Geometry check sheet. Reference: drawing and pictorial views, mm from the part's lowest x, y, z. A direction names the side the tool comes from. Coordinates: 2 decimals unless noted, no trailing zeros. Write each loop counter-clockwise with the first axis right and the second up, starting at its lowest first coordinate (ties: lowest second). Pieces come first, ordered by that corner, then holes. Notation, with made-up numbers: (65.5, 3) -> (95.5, 3) arc R17 cw to (95.5, 16) -> close; hole circle Ø11 at (73.5, 42.25). An arc over 180 degrees is marked (long way). Answer in a Markdown table with one row per item.
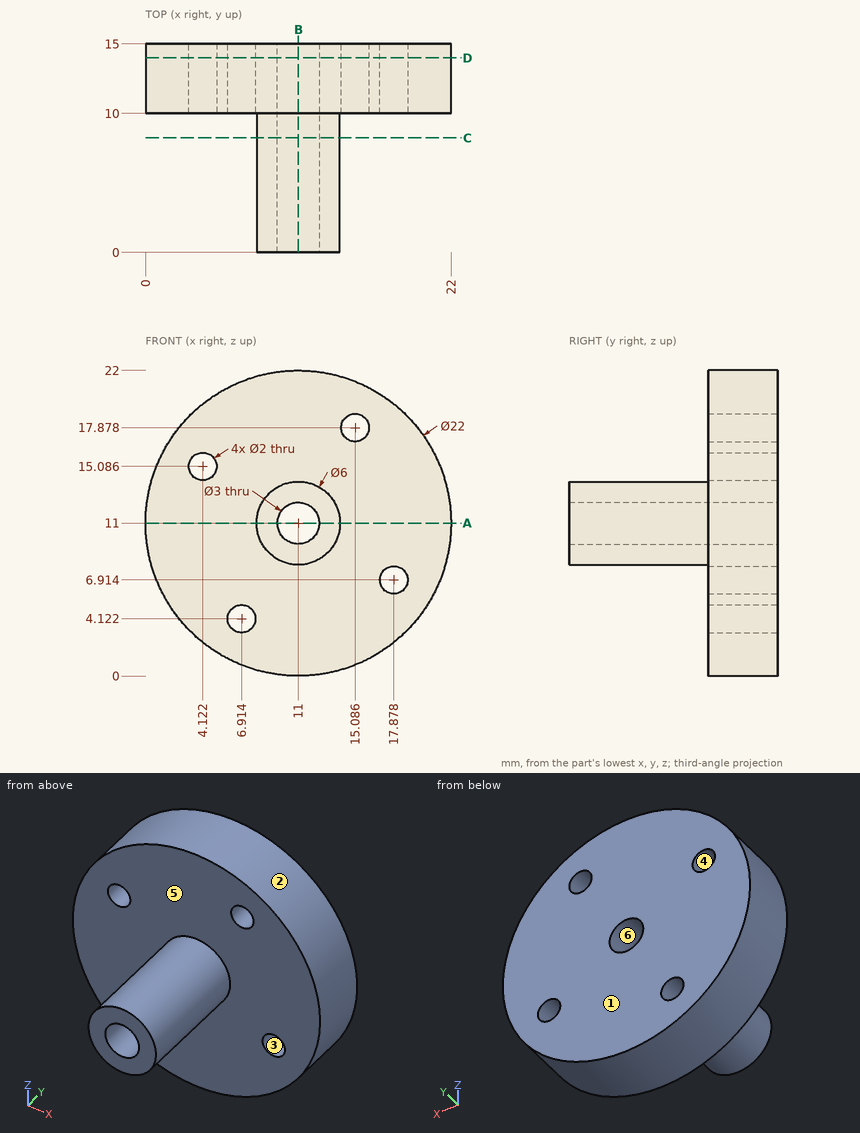
1. Thickness scan on line 1 (Z direction, x = 11, y = 11.75); line 2 (Y direction, x = 1.75, z = 6.5); line 3 (X direction, y = 4.5, z = 11.5) (1 decimal). Record the ranges inside material, lowest first. Write a range as from..to.
Geometry says:
| item | result |
|---|---|
| line 1 | 0..9.5, 12.5..22 |
| line 2 | 10..15 |
| line 3 | 8..9.6, 12.4..14 |
2. Mould release check, pull along X, two halves, no side actions. Record for the marked faces 1, 2, 3 and 4: released by +X, released by -X, zero draft, split by the parting line, or undercut.
Geometry says:
| item | result |
|---|---|
| face 1 | zero draft |
| face 2 | split by the parting line |
| face 3 | undercut |
| face 4 | undercut |
3. Tool access check on the marked faces 5 and 6. Record the directions out of +Z, -Z, +X, -X, +Y, -Y that give a thin tool (end or side, any length) a straight path to the whole face; none if there is none.
Geometry says:
| item | result |
|---|---|
| face 5 | -Y |
| face 6 | +Y, -Y |
4. Depth check by flat-ended pin: P1, Ø3, axis at y = 12, z = 13.5, coming from the +X side; P2, Ø2.5, axis at x = 6.91, z = 4.12, coming from the -Y side; P3, Ø1.5, axis at y = 4, z = 13, coming from the -X side. Enter the tip coordinate at first touch or a pass-through.
Geometry says:
| item | result |
|---|---|
| P1 | x = 21.95 |
| P2 | y = 10 |
| P3 | x = 8.27 |
5. Section check D-D, the plane y = 14. Record the boundary of the cut face in (x, z).
Geometry says:
| item | result |
|---|---|
| outline | circle Ø22 at (11, 11); hole circle Ø2 at (4.12, 15.09); hole circle Ø2 at (6.91, 4.12); hole circle Ø3 at (11, 11); hole circle Ø2 at (15.09, 17.88); hole circle Ø2 at (17.88, 6.91) |
6. Section check C-C, the plane y = 8.25. Record the boundary of the cut face in (x, z).
Geometry says:
| item | result |
|---|---|
| outline | circle Ø6 at (11, 11); hole circle Ø3 at (11, 11) |
7. Section check A-A, the plane z = 11. Record the boundary of the cut face in (x, y).
Geometry says:
| item | result |
|---|---|
| outline | (0, 10) -> (8, 10) -> (8, 0) -> (9.5, 0) -> (9.5, 15) -> (0, 15) -> close; (12.5, 0) -> (14, 0) -> (14, 10) -> (22, 10) -> (22, 15) -> (12.5, 15) -> close |
8. Section check B-B, the plane x = 11. Record the boundary of the cut face in (y, z).
Geometry says:
| item | result |
|---|---|
| outline | (0, 8) -> (10, 8) -> (10, 0) -> (15, 0) -> (15, 9.5) -> (0, 9.5) -> close; (0, 12.5) -> (15, 12.5) -> (15, 22) -> (10, 22) -> (10, 14) -> (0, 14) -> close |
